Verification items for the finished model (mm, model axes). Face numbers are marked on the shaded views. A direction names the side the tool comes from. Round coordinates to 2 decimals unless told otherwise and drop trailing zeros. Write each loop counter-clockwise with the first axis right and the second up, starting at its lowest first coordinate (ties: lowest second). Pieces come first, ordered by that corner, then holes.
from build123d import *

# Parameters (mm, degrees)
F0_W      = 64.756296
F0_H      = 64.756296
F1_DEPTH  = 53.34
F1_FACE_W = 64.756296
F1_FACE_H = 64.756296
F2_DEPTH  = 53.34
F3_SIZE   = 12.7
F4_SIZE   = 12.7
F5_SIZE   = 12.7
F6_SIZE   = 12.7
F7_T      = -2.54


with BuildPart() as f1:
    # F0 (on Top) → F1 (new body)
    with BuildSketch(Plane.XY):
        Rectangle(F0_W, F0_H)
    extrude(amount=F1_DEPTH)

    # F1_face (on face) → F2 (join)
    with BuildSketch(Plane(origin=(0, 0, 0), x_dir=(1, 0, 0), z_dir=(0, 0, -1))):
        Rectangle(F1_FACE_W, F1_FACE_H)
    extrude(amount=F2_DEPTH)

    # F3
    f3_edges = [f1.edges().sort_by_distance(p)[0] for p in [
        (-32.378148, -32.378148, 0),
    ]]
    chamfer(f3_edges, length=F3_SIZE)

    # F4
    f4_edges = [f1.edges().sort_by_distance(p)[0] for p in [
        (-32.378148, 32.378148, 0),
    ]]
    chamfer(f4_edges, length=F4_SIZE)

    # F5
    f5_edges = [f1.edges().sort_by_distance(p)[0] for p in [
        (32.378148, 32.378148, 0),
    ]]
    chamfer(f5_edges, length=F5_SIZE)

    # F6
    f6_edges = [f1.edges().sort_by_distance(p)[0] for p in [
        (32.378148, -32.378148, 0),
    ]]
    chamfer(f6_edges, length=F6_SIZE)

    # F7
    f7_openings = [f1.faces().sort_by_distance(p)[0] for p in [
        (0, 0, 53.34),
    ]]
    offset(amount=F7_T, openings=f7_openings)


solid = f1.part
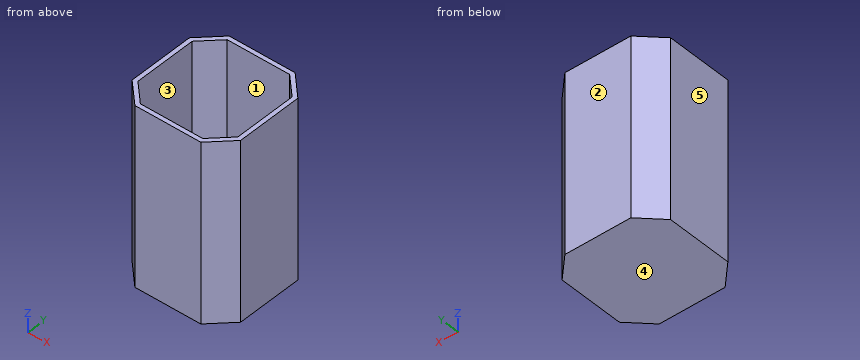
Q1. Sectioned sample at B-B (z = 25.5). Enter the section's corners in (x, y).
Recorded:
outline: (-32.38, -19.68) - (-19.68, -32.38) - (19.68, -32.38) - (32.38, -19.68) - (32.38, 19.68) - (19.68, 32.38) - (-19.68, 32.38) - (-32.38, 19.68) - close; hole (-29.84, -18.63) - (-18.63, -29.84) - (18.63, -29.84) - (29.84, -18.63) - (29.84, 18.63) - (18.63, 29.84) - (-18.63, 29.84) - (-29.84, 18.63) - close
Q2. Release check for a two-part mould opening along X. For the marked faces 3, 4 and 5 record: released by +X, released by -X, zero draft, split by the parting line, or undercut.
Recorded:
face 3: undercut
face 4: zero draft
face 5: released by -X
Q3. Material ranges on line 1 along Y through (x, z) = (0, 37.5); line 2 along Z through (x, y) = (27.5, -9), recorded low to high.
Recorded:
line 1: y = -32.38 to -29.84, 29.84 to 32.38
line 2: z = -53.34 to -50.8
Q4. Sectioned sample at A-A (y = -5.5). Enter the section's corners in (x, z), plus the area to 3 significant figures.
Recorded:
outline: (-32.38, -53.34) - (32.38, -53.34) - (32.38, 53.34) - (29.84, 53.34) - (29.84, -50.8) - (-29.84, -50.8) - (-29.84, 53.34) - (-32.38, 53.34) - close
area: 694 mm2
Q5. Tool access check on the marked faces 1 and 2. Record the directions out of +Z, -Z, +X, -X, +Y, -Y that give a thin tool (end or side, any length) a straight path to the whole face; none if there is none.
Recorded:
face 1: +Z
face 2: +Z, -Z, +X, -X, +Y
Q6. Depth check by flat-ended pin: P1, Ø18, axis at x = 0, y = 5, coming from the +Z side. Enter the tip coordinate at first touch or a pass-through.
Recorded:
P1: stops at z = -50.8
